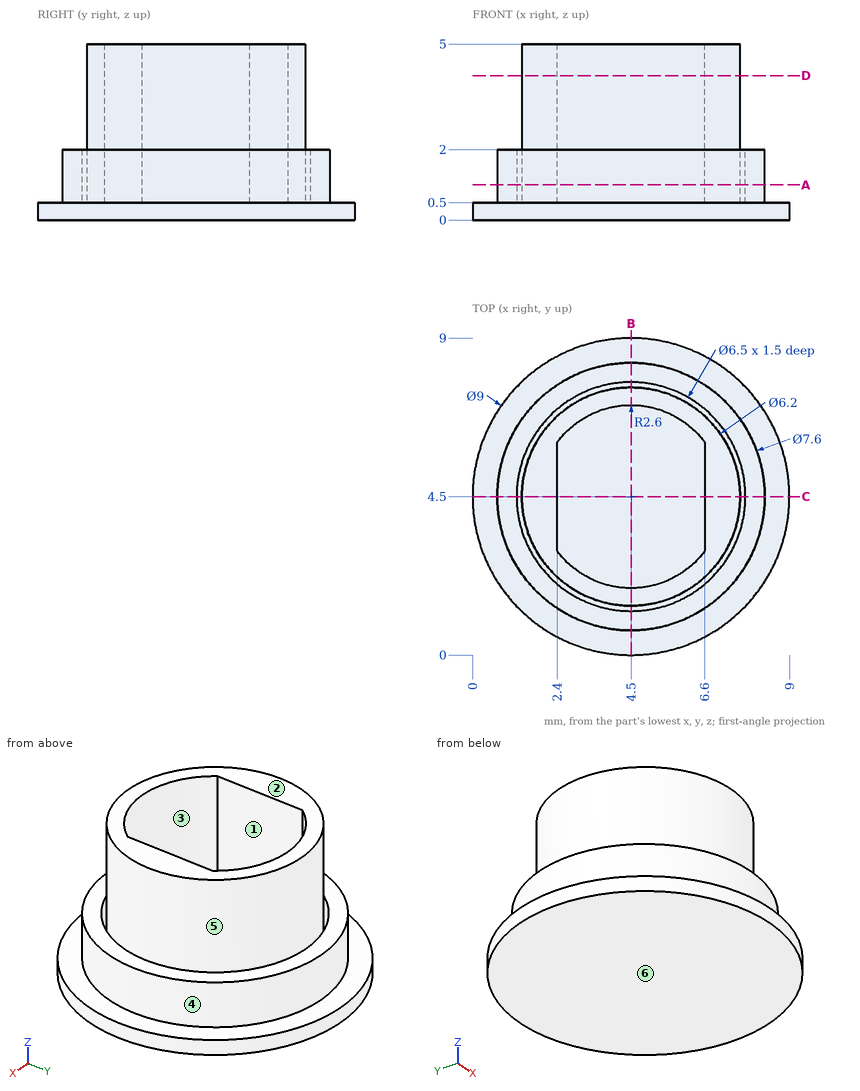
Source: three-view drawing plus pictorial views. Frame: mm from the lowest corner of the part. A direction names the side the tool comes from. Round coordinates to 2 decimals unless told otherwise and drop trailing zeros. Loops run counter-clockwise (first coordinate to the right, second up) from the corner with the lowest first, then second, coordinate; pieces in that order, holes last. Notation, with made-up numbers: M -15,-18.75 L 27,-18.75 A19 ccw 27,14.25 Z; hole C 70,48.25 d10. An arc over 180 degrees is marked long. Put each result on its own line as item: value. Start each with the question number.
(1) Section query C-C (y = 4.5). Return loops of the section in (x, z), then the cut area to 4 significant figures.
(2) Draft query along Y for the marked faces 3, 4, 5 and 6. Return one class per face: +Y half, -Y half, draft (parallel to the pull), parting line (faces both ways), or undercut.
(3) Set-up query: the marked faces 1 and 2. Return all of +Z, -Z, +X, -X, +Y, -Y with unobstructed straight access to the full face (end or side cutting, diameter ignored); none if empty.
(4) Section query B-B (x = 4.5). Return loops of the section in (y, z).
(5) Contact query for flat-ended pins moving along their axis: pin 1 Ø2 at (x, z) = (4.5, 2.5) entering from -Y; pin 2 Ø2.5 at (y, z) = (4, 2) entering from -X; pin 3 Ø2.5 at (x, y) = (4, 5.5) entering from +Z. Output: stop coordinate, or through.
(6) Material intervals for line 1 along X through (y, z) = (5.25, 1.1); line 2 along X through (y, z) = (4.5, 3.15); line 3 along Y through (x, z) = (4.75, 1.4), sorted ascending. Write a range as [from, to].
(7) Section query D-D (z = 4.1). Return loops of the section in (x, y).
(8) Section query A-A (z = 1). Return loops of the section in (x, y), then the cut area to 3 significant figures.
Findings below:
1. outline: M 0,0 L 9,0 L 9,0.5 L 8.3,0.5 L 8.3,2 L 7.75,2 L 7.75,0.5 L 7.6,0.5 L 7.6,5 L 6.6,5 L 6.6,0.5 L 2.4,0.5 L 2.4,5 L 1.4,5 L 1.4,0.5 L 1.25,0.5 L 1.25,2 L 0.7,2 L 0.7,0.5 L 0,0.5 Z
1. area: 15.15 mm2
2. face 3: undercut
2. face 4: parting line
2. face 5: undercut
2. face 6: draft
3. face 1: +Z
3. face 2: +Z, +X, -X, +Y, -Y
4. outline: M 0,0 L 9,0 L 9,0.5 L 8.3,0.5 L 8.3,2 L 7.75,2 L 7.75,0.5 L 7.6,0.5 L 7.6,5 L 7.1,5 L 7.1,0.5 L 1.9,0.5 L 1.9,5 L 1.4,5 L 1.4,0.5 L 1.25,0.5 L 1.25,2 L 0.7,2 L 0.7,0.5 L 0,0.5 Z
5. pin 1: stops at y = 0.7
5. pin 2: stops at x = 0.7
5. pin 3: stops at z = 0.5
6. line 1: x = [0.77, 1.34], [1.49, 2.4], [6.6, 7.51], [7.66, 8.23]
6. line 2: x = [1.4, 2.4], [6.6, 7.6]
6. line 3: y = [0.71, 1.26], [1.41, 1.91], [7.09, 7.59], [7.74, 8.29]
7. outline: C 4.5,4.5 d6.2; hole M 2.4,2.97 A2.6 ccw 6.6,2.97 L 6.6,6.03 A2.6 ccw 2.4,6.03 Z
8. outline: C 4.5,4.5 d7.6; C 4.5,4.5 d6.2; hole C 4.5,4.5 d6.5; hole M 2.4,2.97 A2.6 ccw 6.6,2.97 L 6.6,6.03 A2.6 ccw 2.4,6.03 Z
8. area: 23.2 mm2
